```python
from build123d import *

# Parameters (mm, degrees)
BOSS_EXTRUDE1_DEPTH = 3
SKETCH2_R           = 7
SKETCH2_R_2         = 2.65
CUT_EXTRUDE1_DEPTH  = 3
FILLET1_R           = 10


with BuildPart() as part:
    # Sketch1 → Boss-Extrude1 (new body)
    with BuildSketch(Plane.XY):
        Polygon((0, 0), (51.961524227, 90), (201.961524227, 90), (150, 0), align=None)
    extrude(amount=BOSS_EXTRUDE1_DEPTH)

    # Sketch2 → Cut-Extrude1 (cut)
    with BuildSketch(Plane.XY.offset(3)):
        with Locations((23, 12)):
            Circle(SKETCH2_R)
        with Locations((108, 30)):
            Circle(SKETCH2_R_2)
        with Locations((61.961524227, 80)):
            Circle(SKETCH2_R_2)
        with Locations((181.961524227, 80)):
            Circle(SKETCH2_R_2)
    extrude(amount=-CUT_EXTRUDE1_DEPTH, mode=Mode.SUBTRACT)

    # Fillet1
    fillet1_edges = [part.edges().sort_by_distance(p)[0] for p in [
        (0, 0, 1.5),
        (51.961524227, 90, 1.5),
        (201.961524227, 90, 1.5),
        (150, 0, 1.5),
    ]]
    fillet(fillet1_edges, radius=FILLET1_R)


solid = part.part
```
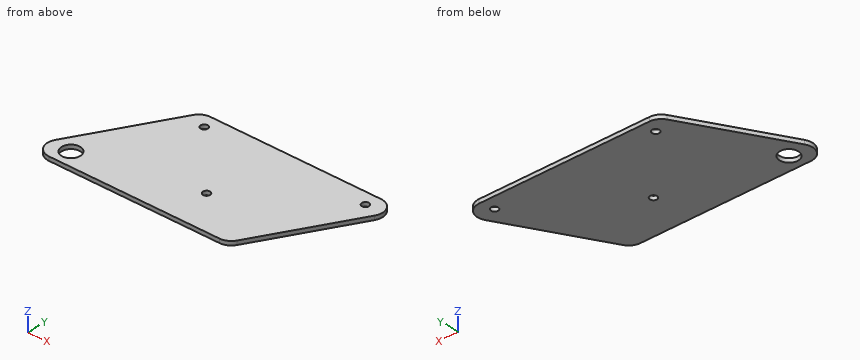
Geometry: final body of the model. Coordinates: model frame, mm. Coordinates: 2 decimals unless noted, no trailing zeros. Order: outer loops, then holes, each group sorted by start corner. A loop starts at its lowest first (then second) coordinate and runs counter-clockwise, first axis right, second up. Notation, with made-up numbers: (51, 63) -> (62, 63) arc R29 ccw to (62, 94) -> close; hole circle Ø2 at (66.5, 28.25). An arc over 180 degrees is marked (long way). Use CSV: the item, a comma, the result in double quotes.
1) Section C-C on y = 30. Output: boundary loops of the cut face in (x, z), then the cut area to 3 significant figures.
Findings:
outline,"(17.32, 0) -> (105.35, 0) -> (105.35, 3) -> (17.32, 3) -> close; (110.65, 0) -> (167.32, 0) -> (167.32, 3) -> (110.65, 3) -> close"
area,"434 mm^2"
2) Line query: line 1 (Y direction, x = 23, z = 0.8); line 2 (X direction, y = 31, z = 1.3); line 3 (Y direction, x = 61, z = 1.2). Output: solid intervals per line, ascending.
Findings:
line 1,"y = 0 to 5, 19 to 39.84"
line 2,"x = 17.9 to 105.55, 110.45 to 167.9"
line 3,"y = 0 to 77.53, 82.47 to 90"
3) Pin query (flat end, axial travel): pin 1 Ø1.5 at (y, z) = (66.5, 2.5) entering from +X; pin 2 Ø5 at (x, y) = (108, 30) entering from -Z; pin 3 Ø2 at (x, y) = (76, 34.5) entering from -Z. Return the tip coordinate at first contact, or that it passes through.
Findings:
pin 1,"stops at x = 188.83"
pin 2,"passes through"
pin 3,"stops at z = 0"
4) Section D-D on y = 80. Output: boundary loops of the cut face in (x, z).
Findings:
outline,"(46.19, 0) -> (59.31, 0) -> (59.31, 3) -> (46.19, 3) -> close; (64.61, 0) -> (179.31, 0) -> (179.31, 3) -> (64.61, 3) -> close; (184.61, 0) -> (194.64, 0) -> (194.64, 3) -> (184.61, 3) -> close"
5) Section B-B on z = 1.6. Output: boundary loops of the cut face in (x, y), then the cut area to 3 significant figures.
Findings:
outline,"(8.66, 15) arc R10 ccw to (17.32, 0) -> (144.23, 0) arc R10 ccw to (152.89, 5) -> (193.3, 75) arc R10 ccw to (184.64, 90) -> (57.74, 90) arc R10 ccw to (49.07, 85) -> close; hole circle Ø14 at (23, 12); hole circle Ø5.3 at (61.96, 80); hole circle Ø5.3 at (108, 30); hole circle Ø5.3 at (181.96, 80)"
area,"13,100 mm^2"
6) Section A-A on x = 108. Output: boundary loops of the cut face in (y, z).
Findings:
outline,"(0, 0) -> (27.35, 0) -> (27.35, 3) -> (0, 3) -> close; (32.65, 0) -> (90, 0) -> (90, 3) -> (32.65, 3) -> close"
